Design review of the part built by this model. Coordinates are the model's own, in mm. A direction names the side the tool comes from. Round coordinates to 2 decimals unless told otherwise and drop trailing zeros. Order: outer loops, then holes, each group sorted by start corner. A loop starts at its lowest first (then second) coordinate and runs counter-clockwise, first axis right, second up. Notation, with made-up numbers: (83.25, 7.5) - (112.25, 7.5) arc R22 cw to (112.25, 13.5) - close; hole circle Ø8 at (-31.75, 2). An arc over 180 degrees is marked (long way). Answer as a JSON object with one key per item and string values. Group by question number.
from build123d import *

# Parameters (mm, degrees)
F1_DEPTH = 5.08
F2_R     = 4.4958
F3_DEPTH = 1.27
F4_R     = 4.4958
F5_DEPTH = 1.27


with BuildPart() as f1:
    # F0 (on Right) → F1 (new body)
    with BuildSketch(Plane.YZ):
        Polygon((0, 0), (-12.7, 21.997045), (-25.4, 0), align=None)
    extrude(amount=F1_DEPTH)

    # F2 (on face) → F3 (cut)
    with BuildSketch(Plane.YZ.offset(5.08)):
        with Locations((-12.467312, 7.535188)):
            Circle(F2_R)
    extrude(amount=-F3_DEPTH, mode=Mode.SUBTRACT)

    # F4 (on face) → F5 (cut)
    with BuildSketch(Plane(origin=(0, 0, 0), x_dir=(0, -1, 0), z_dir=(-1, 0, 0))):
        with Locations((12.821567, 8.129397)):
            Circle(F4_R)
    extrude(amount=-F5_DEPTH, mode=Mode.SUBTRACT)


solid = f1.part
1. To check wall thickness, follow line 1 (Y direction, x = 2.3, z = 7.5); line 2 (Z direction, x = 2.8, y = -15.5); line 3 (Y direction, x = 4.35, z = 3.75). State the ranges of each line that lie inside material, in increasing order. Write a range as from..to.
2. Take a section at A-A, the plane x = 1.65. Give the boundary of the cut face in (y, z).
3. Take a section at C-C, the plane y = -13.25. Give the boundary of the cut face in (x, z).
4. Tool access review of faces 5 (the flat face through (3, -13, 0)), 6 (the flat face through (1.27, -13, 8)), 7 (the flat face through (3.81, -13, 8)): name each direction out of +Z, -Z, +X, -X, +Y, -Y from which nothing blocks a thin tool from reaching the whole face with its end or side.
5. Take a section at D-D, the plane y = -6. Give the boundary of the cut face in (x, z).
6. Take a section at B-B, the plane z = 11.5. Give the boundary of the cut face in (x, y), then the cut area to 3 significant figures.
7. Mouldability with a two-part tool opening along Z and no side actions: class faces 1 (the cylindrical face through (4.454, -15.781, 10.574)), 2 (the flat face through (5.08, -16, 11)), 3 (the flat face through (2.504, -18.961, 11.153)), 4 (the cylindrical face through (0.626, -16.975, 6.407)) as pulls with the +Z half, pulls with the -Z half, needs draft (parallel to the pull), parting line crosses it, or undercut.
8. Clearance check with flat-ended pins moving along their axes: P1, Ø3, axis at x = 1, z = 8, coming from the +Y side; P2, Ø4.5, axis at y = -13.5, z = 8.5, coming from the -X side; P3, Ø2.5, axis at y = -12, z = 7, coming from the +X side. State where each tip first meets the part, or that it passes through.
Response values:
{
 "1": {"line 1": "-21.07..-4.33", "line 2": "0..17.15", "line 3": "-23.23..-14.89, -10.04..-2.17"},
 "2": {"outline": "(-25.4, 0) - (0, 0) - (-12.7, 22) - close"},
 "3": {"outline": "(0, 0) - (5.08, 0) - (5.08, 3.11) - (3.81, 3.11) - (3.81, 11.96) - (5.08, 11.96) - (5.08, 21.04) - (0, 21.04) - (0, 12.6) - (1.27, 12.6) - (1.27, 3.65) - (0, 3.65) - close"},
 "4": {"face 5": "-Z, +X, -X, +Y, -Y", "face 6": "-X", "face 7": "+X"},
 "5": {"outline": "(0, 0) - (5.08, 0) - (5.08, 10.39) - (0, 10.39) - close"},
 "6": {"outline": "(0, -18.76) - (5.08, -18.76) - (5.08, -14.59) - (3.81, -14.59) - (3.81, -10.35) - (5.08, -10.35) - (5.08, -6.64) - (0, -6.64) - (0, -9.85) - (1.27, -9.85) - (1.27, -15.8) - (0, -15.8) - close", "area": "48.6 mm2"},
 "7": {"face 1": "undercut", "face 2": "needs draft", "face 3": "pulls with the +Z half", "face 4": "undercut"},
 "8": {"P1": "y = -3.75", "P2": "x = 1.27", "P3": "x = 3.81"}
}
